from build123d import *

# Parameters (mm, degrees)
SKETCH1_R           = 2.225
SKETCH1_R_2         = 1.725
SKETCH1_R_3         = 1.225
BOSS_EXTRUDE1_DEPTH = 3
FILLET1_R           = 4


with BuildPart() as part:
    # Sketch1 → Boss-Extrude1 (new body)
    with BuildSketch(Plane.XY):
        with BuildLine():
            Line((3.464101615, -2), (11.417424305, -2))
            ThreePointArc((11.417424305, -2), (20.183300133, -2.738612788), (16, 5))
            Line((16, 5), (7, 5))
            Line((7, 5), (7, 11))
            ThreePointArc((7, 11), (6.121320344, 13.121320344), (4, 14))
            Line((4, 14), (-1, 14))
            ThreePointArc((-1, 14), (-3.121320344, 13.121320344), (-4, 11))
            Line((-4, 11), (-4, 0))
            ThreePointArc((-4, 0), (-1.03527618, -3.863703305), (3.464101615, -2))
        make_face()
        Circle(SKETCH1_R, mode=Mode.SUBTRACT)
        with Locations((16, 0)):
            Circle(SKETCH1_R_2, mode=Mode.SUBTRACT)
        with Locations((-1, 11)):
            Circle(SKETCH1_R_3, mode=Mode.SUBTRACT)
        with Locations((4, 11)):
            Circle(SKETCH1_R_3, mode=Mode.SUBTRACT)
    extrude(amount=BOSS_EXTRUDE1_DEPTH)

    # Fillet1
    fillet1_edges = [part.edges().sort_by_distance(p)[0] for p in [
        (7, 5, 1.5),
    ]]
    fillet(fillet1_edges, radius=FILLET1_R)


solid = part.part
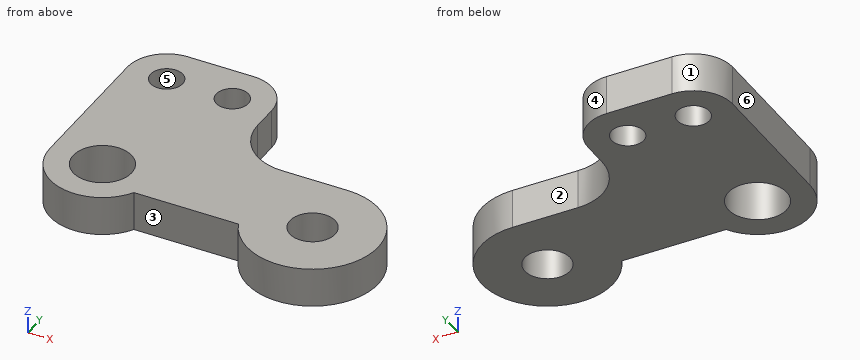
The listing builds one solid part. Answer for the finished solid, in the listing's coordinates (mm). Face numbers are marked on the shaded views. A direction names the side the tool comes from. Round coordinates to 2 decimals unless told otherwise and drop trailing zeros. Order: outer loops, then holes, each group sorted by start corner. A loop starts at its lowest first (then second) coordinate and runs counter-clockwise, first axis right, second up. Notation, with made-up numbers: (73, 45.25) -> (130, 45.25) arc R29 cw to (130, 80.25) -> close; hole circle Ø8 at (-7, 66.25). An arc over 180 degrees is marked (long way). One line per item, written item: value.
Item 1: For the marked faces 1, 2 and 3, determine the directions among +Z, -Z, +X, -X, +Y, -Y from which every point of the face is accessible in a straight line to the end or side of a thin tool.
Taken from the geometry:
face 1: +Z, -Z, -X, +Y
face 2: +Z, -Z, +X, +Y
face 3: +Z, -Z, -Y
Item 2: Find section A-A, the plane z = 1.8. Give the vertices of the cut face in (x, y) (3 decimals), then the cut area to 3 significant figures.
Taken from the geometry:
outline: (-4, 0) arc R4 ccw to (3.464, -2) -> (11.417, -2) arc R5 ccw (long way) to (16, 5) -> (11, 5) arc R4 cw to (7, 9) -> (7, 11) arc R3 ccw to (4, 14) -> (-1, 14) arc R3 ccw to (-4, 11) -> close; hole circle Ø4.45 at (0, 0); hole circle Ø2.45 at (-1, 11); hole circle Ø2.45 at (4, 11); hole circle Ø3.45 at (16, 0)
area: 263 mm2
Item 3: For a pull along X with two mould halves and no side action, classify the marked faces 4, 5 and 6 as released by +X, released by -X, zero draft, split by the parting line, or undercut.
Taken from the geometry:
face 4: released by +X
face 5: undercut
face 6: released by -X
Item 4: Given P1, Ø0.9, axis at x = 13, z = 1.5, coming from the +Y side; P2, Ø1.6, axis at y = 10.5, z = 1.5, coming from the +X side; P3, Ø1.5, axis at x = 13.5, z = 2, coming from the -Y side, each flat-ended and moving along its own axis, determine where each tip first touches the part or whether it passes through.
Taken from the geometry:
P1: stops at y = 5
P2: stops at x = 7
P3: stops at y = -4.68
Item 5: Find section D-D, the plane x = 14. Give the vertices of the cut face in (y, z).
Taken from the geometry:
outline: (-4.58, 0) -> (5, 0) -> (5, 3) -> (-4.58, 3) -> close
Item 6: Find section C-C, the plane x = 9.5. Give the vertices of the cut face in (y, z), then the cut area to 3 significant figures.
Taken from the geometry:
outline: (-2, 0) -> (5.29, 0) -> (5.29, 3) -> (-2, 3) -> close
area: 21.9 mm2
Item 7: Straight lines are drawn through the part: L1, parallel to Y at x = 4, z = 1.05 (3 decimals); L2, parallel to Y at x = -1, z = 2.2 (3 decimals); L3, parallel to X at y = 9.5, z = 0.95. For each, find the intervals that lie inside material, in ascending order.
Taken from the geometry:
L1: y = -2 to 9.775, 12.225 to 14
L2: y = -3.873 to -1.988, 1.988 to 9.775, 12.225 to 14
L3: x = -4 to 7
Item 8: Find section B-B, the plane y = 10.25. Give the vertices of the cut face in (x, z).
Taken from the geometry:
outline: (-4, 0) -> (-1.97, 0) -> (-1.97, 3) -> (-4, 3) -> close; (-0.03, 0) -> (3.03, 0) -> (3.03, 3) -> (-0.03, 3) -> close; (4.97, 0) -> (7, 0) -> (7, 3) -> (4.97, 3) -> close
